from build123d import *

# Parameters (mm, degrees)
SKETCH25_W               = 7
SKETCH25_H               = 8
BOSS_EXTRUDE5_DEPTH      = 12.8
BOSS_EXTRUDE6_DEPTH      = 12
BOSS_EXTRUDE6_DEPTH_BACK = 1.5
SKETCH26_W               = 24
SKETCH26_H               = 8
SKETCH26_R               = 2.65
SKETCH27_R               = 1.55
CUT_EXTRUDE1_DEPTH       = 6.5
FILLET1_R                = 2
BOSS_EXTRUDE8_DEPTH      = 2.5
FILLET2_R                = 1.5
BOSS_EXTRUDE9_START      = 13.5
SKETCH30_R               = 3.2
BOSS_EXTRUDE9_DEPTH      = 13.5
SKETCH31_R               = 2.25
CUT_EXTRUDE2_DEPTH       = 4


with BuildPart() as part:
    # Sketch25 → Boss-Extrude5 (new body)
    with BuildSketch(Plane(origin=(0, 0, 0), x_dir=(-1, 0, 0), z_dir=(0, 1, 0))):
        Rectangle(SKETCH25_W, SKETCH25_H)
    extrude(amount=BOSS_EXTRUDE5_DEPTH)

    # Sketch26 → Boss-Extrude6 (add, two sides: drawn at the far end of the back side and taken through both)
    with BuildSketch(Plane(origin=(0, 0, 0), x_dir=(-1, 0, 0), z_dir=(0, 1, 0)).offset(-BOSS_EXTRUDE6_DEPTH_BACK)):
        Rectangle(SKETCH26_W, SKETCH26_H)
        with Locations(Location((-8, 0, 0), (0, 0, 90))):
            Circle(SKETCH26_R, mode=Mode.SUBTRACT)
        with Locations(Location((8, 0, 0), (0, 0, 90))):
            Circle(SKETCH26_R, mode=Mode.SUBTRACT)
    extrude(amount=BOSS_EXTRUDE6_DEPTH + BOSS_EXTRUDE6_DEPTH_BACK)

    # Sketch27 → Cut-Extrude1 (cut)
    with BuildSketch(Plane(origin=(0, 12.8, 0), x_dir=(1, 0, 0), z_dir=(0, 1, 0))):
        with Locations(Location((0, 0, 0), (0, 0, 270))):
            Circle(SKETCH27_R)
    extrude(amount=-CUT_EXTRUDE1_DEPTH, mode=Mode.SUBTRACT)

    # Fillet1
    fillet1_edges = [part.edges().sort_by_distance(p)[0] for p in [
        (12, 5.25, 4),
        (-12, 5.25, -4),
        (12, 5.25, -4),
        (-12, 5.25, 4),
    ]]
    fillet(fillet1_edges, radius=FILLET1_R)

    # Sketch29 → Boss-Extrude8 (add)
    with BuildSketch(Plane.XZ.offset(1.5)):
        with BuildLine():
            Line((-17.090822427, -3.57750922), (-12, 0.816317906))
            Line((-12, 0.816317906), (-10.745987583, -2.422706372))
            Line((-10.745987583, -2.422706372), (-7.78514456, -4))
            Line((-7.78514456, -4), (-12.909177573, -8.42249078))
            ThreePointArc((-12.909177573, -8.42249078), (-17.42249078, -8.090822427), (-17.090822427, -3.57750922))
        make_face()
        with BuildLine():
            Line((17.090822427, -3.57750922), (12, 0.816317906))
            Line((12, 0.816317906), (10.79122124, -2.606916283))
            Line((10.79122124, -2.606916283), (7.78514456, -4))
            Line((7.78514456, -4), (12.909177573, -8.42249078))
            ThreePointArc((12.909177573, -8.42249078), (17.42249078, -8.090822427), (17.090822427, -3.57750922))
        make_face()
    extrude(amount=-BOSS_EXTRUDE8_DEPTH)

    # Fillet2
    fillet2_edges = [part.edges().sort_by_distance(p)[0] for p in [
        (8.89257228, 1, -4),
        (-11.414213562, 1, -3.414213562),
        (-8.89257228, 1, -4),
        (-12, -0.25, 0.816317906),
        (-7.78514456, -0.25, -4),
        (-12, 1, -0.591841047),
        (11.414213562, 1, -3.414213562),
        (12, 1, -0.591841047),
        (7.78514456, -0.25, -4),
        (12, -0.25, 0.816317906),
    ]]
    fillet(fillet2_edges, radius=FILLET2_R)

    # Sketch30 → Boss-Extrude9 (add)
    with BuildSketch(Plane.XZ.offset(1.5).offset(BOSS_EXTRUDE9_START)):
        with Locations(Location((-15, -6, 0), (0, 0, 270))):
            Circle(SKETCH30_R)
        with Locations(Location((15, -6, 0), (0, 0, 270))):
            Circle(SKETCH30_R)
    extrude(amount=-BOSS_EXTRUDE9_DEPTH)

    # Sketch31 → Cut-Extrude2 (cut)
    with BuildSketch(Plane.XZ.offset(15)):
        with Locations(Location((-15, -6, 0), (0, 0, 270))):
            Circle(SKETCH31_R)
        with Locations(Location((15, -6, 0), (0, 0, 270))):
            Circle(SKETCH31_R)
    extrude(amount=-CUT_EXTRUDE2_DEPTH, mode=Mode.SUBTRACT)


solid = part.part
Work out the finished part from the listing and answer in its coordinate system (mm). A direction names the side the tool comes from. Give positions to 0.01 mm unless a question says otherwise; leave off trailing zeros. Loops run counter-clockwise (first coordinate to the right, second up) from the corner with the lowest first, then second, coordinate; pieces in that order, holes last. Notation, with made-up numbers: (-38.5, 6.25) -> (-31.5, 6.25) arc R27 ccw to (-31.5, 42.25) -> close; hole circle Ø2 at (-19.5, 67). An arc over 180 degrees is marked (long way). Use a Markdown table: item, result. Add a question column.
1. Section B-B on y = -2.5 is taken. Determine the outline of the cut face in (x, z).
2. Section C-C on x = -15 is taken. Determine the outline of the cut face in (y, z).
3. Determine the mould class of faces 6 (the flat face through (0, 6, -4)), 7 (the flat face through (-15, 1, -6)), 8 (the cylindrical face through (0.466, 9.596, 1.478)) for opening direction Z: released by +Z, released by -Z, zero draft, split by the parting line, or undercut.
4. Find the intervals of material crossed by probe 1 along X at (y, z) = (-13.1, -6); probe 2 along X at (y, z) = (7.25, 0); probe 3 along X at (y, z) = (4.25, -0.5), in increasing order.
5. Flat-ended cylindrical pins translate along their axes: pin 1 Ø2.5 at (x, z) = (-0.5, 0.5) entering from +Y; pin 2 Ø4 at (x, z) = (-10, -1) entering from +Y; pin 3 Ø2 at (y, z) = (8, 0.5) entering from +X; pin 4 Ø1.5 at (x, z) = (12.5, -7.5) entering from +Y. Find the tip coordinate at first contact, or state that the pin passes through.
6. For faces 1 (the flat face through (6, 12, 2)), 2 (the cylindrical face through (-7.757, 0.084, -4.097)), 3 (the flat face through (-15, -11, -6)), 4 (the cylindrical face through (11.43, 7.32, -3.4)), 5 (the flat face through (-6, 12, 2)), determine the directions among +Z, -Z, +X, -X, +Y, -Y from which every point of the face is accessible in a straight line to the end or side of a thin tool.
7. Section A-A on z = -6.5 is taken. Determine the outline of the cut face in (x, y), and give its area (3 significant figures).
Results below:
| question | item | result |
|---|---|---|
| 1 | outline | circle Ø6.4 at (-15, -6); circle Ø6.4 at (15, -6) |
| 2 | outline | (-15, -9.2) -> (1, -9.2) -> (1, -1.77) -> (-1.5, -1.77) -> (-1.5, -2.8) -> (-15, -2.8) -> (-15, -3.75) -> (-11, -3.75) -> (-11, -8.25) -> (-15, -8.25) -> close |
| 3 | face 6 | released by -Z |
| 3 | face 7 | zero draft |
| 3 | face 8 | undercut |
| 4 | probe 1 | x = -18.2 to -17.25, -12.75 to -11.8, 11.8 to 12.75, 17.25 to 18.2 |
| 4 | probe 2 | x = -12 to -10.65, -5.35 to -1.55, 1.55 to 5.35, 10.65 to 12 |
| 4 | probe 3 | x = -12 to -10.6, -5.4 to 5.4, 10.6 to 12 |
| 5 | pin 1 | stops at y = 12.8 |
| 5 | pin 2 | stops at y = 12 |
| 5 | pin 3 | stops at x = 12 |
| 5 | pin 4 | stops at y = 1 |
| 6 | face 1 | +Z, -Z, +X, +Y |
| 6 | face 2 | -Z, +Y, -Y |
| 6 | face 3 | -Y |
| 6 | face 4 | -Z, +X, +Y |
| 6 | face 5 | +Z, -Z, -X, +Y |
| 7 | outline | (-18.16, -15) -> (-17.19, -15) -> (-17.19, -11) -> (-12.81, -11) -> (-12.81, -15) -> (-11.84, -15) -> (-11.84, -1.5) -> (-10.68, -1.5) -> (-10.68, 1) -> (-18.16, 1) -> close; (10.68, -1.5) -> (11.84, -1.5) -> (11.84, -15) -> (12.81, -15) -> (12.81, -11) -> (17.19, -11) -> (17.19, -15) -> (18.16, -15) -> (18.16, 1) -> (10.68, 1) -> close |
| 7 | area | 173 mm^2 |
